Design review of the part shown in the three views and the two pictorial views. Dimensions are in mm from the part's minimum x, y and z. A direction names the side the tool comes from. Round coordinates to 2 decimals unless told otherwise and drop trailing zeros. Order: outer loops, then holes, each group sorted by start corner. A loop starts at its lowest first (then second) coordinate and runs counter-clockwise, first axis right, second up. Notation, with made-up numbers: (22.5, 35) - (65.5, 35) arc R22 cw to (65.5, 51) - close; hole circle Ø9 at (50, -39). An arc over 180 degrees is marked (long way). One line per item, written item: value.
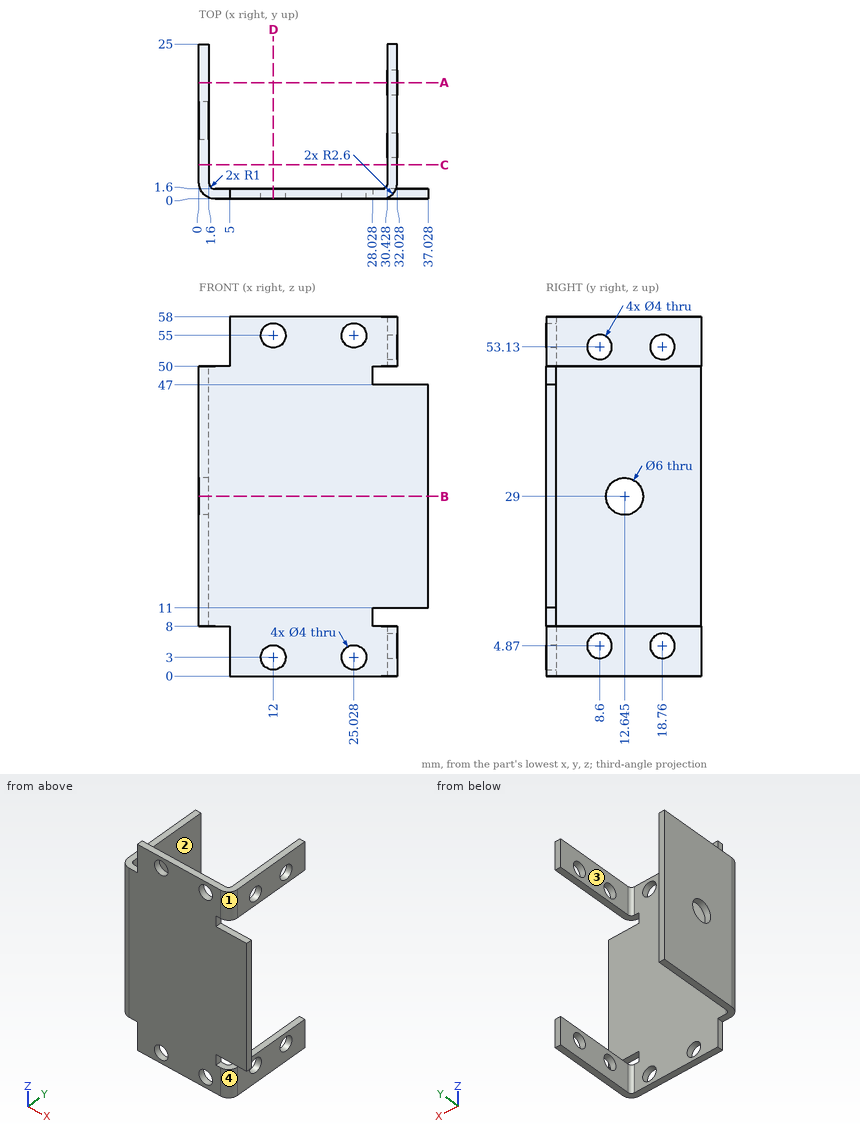
Item 1: Take a section at D-D (x = 12). Write out the cut boundary in (y, z).
Returned:
outline: (0, 0) - (1.6, 0) - (1.6, 1) - (0, 1) - close; (0, 5) - (1.6, 5) - (1.6, 53) - (0, 53) - close; (0, 57) - (1.6, 57) - (1.6, 58) - (0, 58) - close
Item 2: Machinability: for the marked faces 1, 2, 3 and 4, which of the approach directions +Z, -Z, +X, -X, +Y, -Y give a long, thin tool a straight path to every point of the face, cutting with its end or side? Answer none if there is none.
Returned:
face 1: +Z, +X, -Y
face 2: +Z, -Z, +X, +Y
face 3: +Z, -Z, -X, +Y
face 4: -Z, +X, -Y
Item 3: Take a section at C-C (y = 5.5). Write out the cut boundary in (x, z).
Returned:
outline: (0, 8) - (1.6, 8) - (1.6, 50) - (0, 50) - close; (30.43, 0) - (32.03, 0) - (32.03, 8) - (30.43, 8) - close; (30.43, 50) - (32.03, 50) - (32.03, 58) - (30.43, 58) - close
Item 4: Take a section at B-B (z = 29). Write out the cut boundary in (x, y) (1 decimal).
Returned:
outline: (0, 2.6) arc R2.6 ccw to (2.6, 0) - (37, 0) - (37, 1.6) - (2.6, 1.6) arc R1 cw to (1.6, 2.6) - (1.6, 9.6) - (0, 9.6) - close; (0, 15.6) - (1.6, 15.6) - (1.6, 25) - (0, 25) - close
Item 5: Wall thickness on line 1 (Z direction, x = 31.55, y = 8.6); line 2 (X direction, y = 0.3, z = 3) (1 decimal); line 3 (X direction, y = 0.8, z = 55) (1 decimal): over which ranges is each line inside the solid? List them lowest first.
Returned:
line 1: 0 to 2.87, 6.87 to 8, 50 to 51.13, 55.13 to 58
line 2: 5 to 10, 14 to 23, 27 to 30.6
line 3: 5 to 10, 14 to 23, 27 to 31.3
Item 6: For P1, Ø4, axis at y = 15.5, z = 19.5, coming from the +X side; P2, Ø0.5, axis at x = 33, y = 1, coming from the -Z side; P3, Ø4, axis at x = 1.5, y = 6.5, coming from the +Z side, all flat-tipped, find the tip position at first contact; note any pin that passes through.
Returned:
P1: x = 1.6
P2: z = 11
P3: z = 50
Item 7: Take a section at A-A (y = 18.76). Write out the cut boundary in (x, z).
Returned:
outline: (0, 8) - (1.6, 8) - (1.6, 50) - (0, 50) - close; (30.43, 0) - (32.03, 0) - (32.03, 2.87) - (30.43, 2.87) - close; (30.43, 6.87) - (32.03, 6.87) - (32.03, 8) - (30.43, 8) - close; (30.43, 50) - (32.03, 50) - (32.03, 51.13) - (30.43, 51.13) - close; (30.43, 55.13) - (32.03, 55.13) - (32.03, 58) - (30.43, 58) - close
